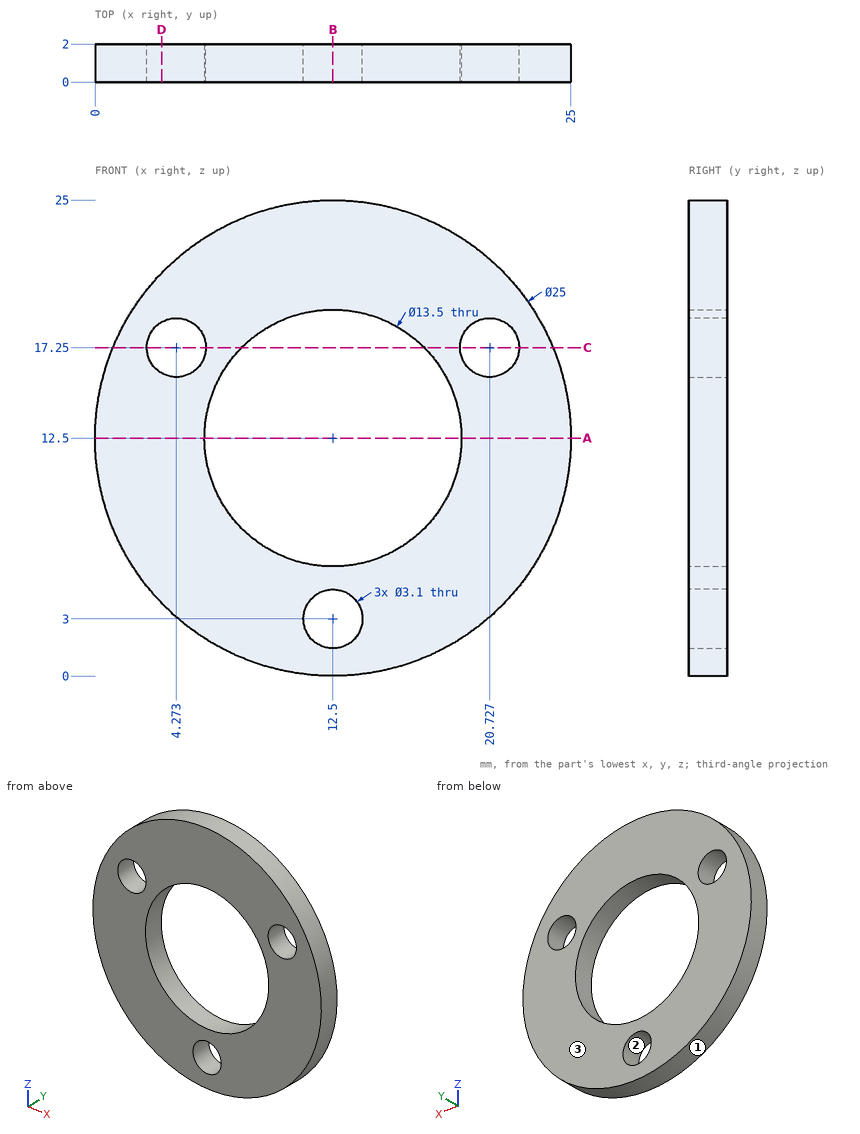
Verification items for this drawing (mm, ordinates from the low corner). Coordinates: 2 decimals unless noted, no trailing zeros. Order: outer loops, then holes, each group sorted by start corner. A loop starts at its lowest first (then second) coordinate and runs counter-clockwise, first axis right, second up. Notation, with made-up numbers: M -17.75,-20 L 29.25,-20 A13 cw 29.25,-3 Z; hole C -35.75,-27 d9. An arc over 180 degrees is marked long. Write each question's results on one line, items separated by ' | '.
1) Section check D-D on x = 3.5. Record the cut outline in (y, z) (1 decimal).
Solved:
outline: M 0,3.8 L 2,3.8 L 2,15.9 L 0,15.9 Z; M 0,18.6 L 2,18.6 L 2,21.2 L 0,21.2 Z
2) Section check B-B on x = 12.5. Record the cut outline in (y, z), plus the area to 3 significant figures.
Solved:
outline: M 0,0 L 2,0 L 2,1.45 L 0,1.45 Z; M 0,4.55 L 2,4.55 L 2,5.75 L 0,5.75 Z; M 0,19.25 L 2,19.25 L 2,25 L 0,25 Z | area: 16.8 mm²
3) Section check A-A on z = 12.5. Record the cut outline in (x, y), plus the area to 3 significant figures.
Solved:
outline: M 0,0 L 5.75,0 L 5.75,2 L 0,2 Z; M 19.25,0 L 25,0 L 25,2 L 19.25,2 Z | area: 23.0 mm²
4) Release check for a two-part mould opening along Z. For the marked faces 1, 2 and 3 record: pulls with the +Z half, pulls with the -Z half, needs draft (parallel to the pull), parting line crosses it, or undercut.
Solved:
face 1: parting line crosses it | face 2: undercut | face 3: needs draft
5) Scan lines: line 1 along X through (y, z) = (0.6, 12.5); line 2 along X through (y, z) = (0.45, 17.25) (1 decimal); line 3 along Z through (x, y) = (11.5, 0.5) (1 decimal). Record each from-to range of solid material in increasing order. Write a range as [from, to].
Solved:
line 1: x = [0, 5.75], [19.25, 25] | line 2: x = [0.9, 2.7], [5.8, 7.7], [17.3, 19.2], [22.3, 24.1] | line 3: z = [0, 1.8], [4.2, 5.8], [19.2, 25]
6) Section check C-C on z = 17.25. Record the cut outline in (x, y).
Solved:
outline: M 0.94,0 L 2.72,0 L 2.72,2 L 0.94,2 Z; M 5.82,0 L 7.7,0 L 7.7,2 L 5.82,2 Z; M 17.3,0 L 19.18,0 L 19.18,2 L 17.3,2 Z; M 22.28,0 L 24.06,0 L 24.06,2 L 22.28,2 Z
7) Gauge pin test, flat ends, axial feed: pin 1 Ø8 at (x, z) = (12.5, 12.5) entering from +Y; pin 2 Ø1 at (x, y) = (3.5, 0.5) entering from +Z (1 decimal). Record the tip position at first contact, or that the pin passes through.
Solved:
pin 1: passes through | pin 2: stops at z = 21.7
